Could you check a few things on this model? Use its own coordinates, in mm. Give positions to 0.01 mm unless a question says otherwise; leave off trailing zeros. Write each question's results on one line, items separated by ' | '. Start each with the question number.
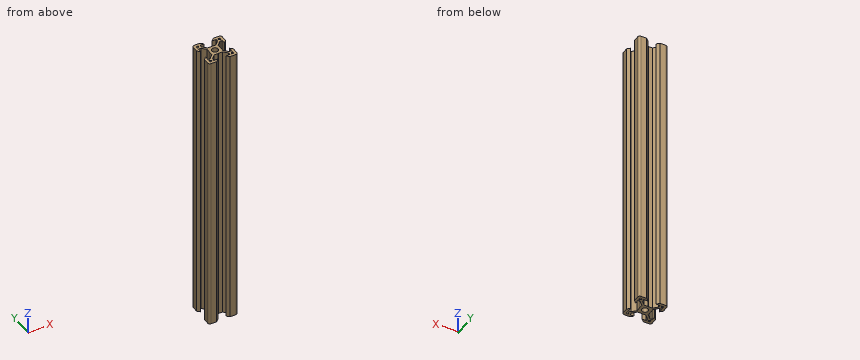
from build123d import *

# Parameters (mm, degrees)
F1_DEPTH = 200


with BuildPart() as f1:
    # F0 (on Top) → F1 (new body)
    with BuildSketch(Plane.XY):
        with BuildLine():
            Line((0, -3.729949), (0, -2.1))
            ThreePointArc((0, -2.1), (-1.484924, -1.484924), (-2.1, 0))
            Line((-2.1, 0), (-3.729949, 0))
            ThreePointArc((-3.729949, 0), (-3.759239, -0.070711), (-3.829949, -0.1))
            Line((-3.829949, -0.1), (-3.829949, -2.84))
            Line((-3.829949, -2.84), (-6.56, -5.570051))
            Line((-6.56, -5.570051), (-8.2, -5.570051))
            Line((-8.2, -5.570051), (-8.2, -2.84))
            Line((-8.2, -2.84), (-10, -4.64))
            Line((-10, -4.64), (-10, -8.5))
            ThreePointArc((-10, -8.5), (-9.56066, -9.56066), (-8.5, -10))
            Line((-8.5, -10), (-4.64, -10))
            Line((-4.64, -10), (-2.84, -8.2))
            Line((-2.84, -8.2), (-5.570051, -8.2))
            Line((-5.570051, -8.2), (-5.570051, -6.56))
            Line((-5.570051, -6.56), (-2.84, -3.829949))
            Line((-2.84, -3.829949), (-0.1, -3.829949))
            ThreePointArc((-0.1, -3.829949), (-0.070711, -3.759239), (0, -3.729949))
        make_face()
        Polygon((-7.780051, -6.640051), (-6.640051, -7.780051), (-6.640051, -8.2), (-8.2, -8.2), (-8.2, -6.640051), align=None, mode=Mode.SUBTRACT)
        with BuildLine():
            ThreePointArc((-2.1, 0), (-1.484924, 1.484924), (0, 2.1))
            Line((0, 2.1), (0, 3.729949))
            ThreePointArc((0, 3.729949), (-0.070711, 3.759239), (-0.1, 3.829949))
            Line((-0.1, 3.829949), (-2.84, 3.829949))
            Line((-2.84, 3.829949), (-5.570051, 6.56))
            Line((-5.570051, 6.56), (-5.570051, 8.2))
            Line((-5.570051, 8.2), (-2.84, 8.2))
            Line((-2.84, 8.2), (-4.64, 10))
            Line((-4.64, 10), (-8.5, 10))
            ThreePointArc((-8.5, 10), (-9.56066, 9.56066), (-10, 8.5))
            Line((-10, 8.5), (-10, 4.64))
            Line((-10, 4.64), (-8.2, 2.84))
            Line((-8.2, 2.84), (-8.2, 5.570051))
            Line((-8.2, 5.570051), (-6.56, 5.570051))
            Line((-6.56, 5.570051), (-3.829949, 2.84))
            Line((-3.829949, 2.84), (-3.829949, 0.1))
            ThreePointArc((-3.829949, 0.1), (-3.759239, 0.070711), (-3.729949, 0))
            Line((-3.729949, 0), (-2.1, 0))
        make_face()
        Polygon((-6.640051, 7.780051), (-7.780051, 6.640051), (-8.2, 6.640051), (-8.2, 8.2), (-6.640051, 8.2), align=None, mode=Mode.SUBTRACT)
        with BuildLine():
            Line((3.729949, 0), (2.1, 0))
            ThreePointArc((2.1, 0), (1.484924, -1.484924), (0, -2.1))
            Line((0, -2.1), (0, -3.729949))
            ThreePointArc((0, -3.729949), (0.070711, -3.759239), (0.1, -3.829949))
            Line((0.1, -3.829949), (2.84, -3.829949))
            Line((2.84, -3.829949), (5.570051, -6.56))
            Line((5.570051, -6.56), (5.570051, -8.2))
            Line((5.570051, -8.2), (2.84, -8.2))
            Line((2.84, -8.2), (4.64, -10))
            Line((4.64, -10), (8.5, -10))
            ThreePointArc((8.5, -10), (9.56066, -9.56066), (10, -8.5))
            Line((10, -8.5), (10, -4.64))
            Line((10, -4.64), (8.2, -2.84))
            Line((8.2, -2.84), (8.2, -5.570051))
            Line((8.2, -5.570051), (6.56, -5.570051))
            Line((6.56, -5.570051), (3.829949, -2.84))
            Line((3.829949, -2.84), (3.829949, -0.1))
            ThreePointArc((3.829949, -0.1), (3.759239, -0.070711), (3.729949, 0))
        make_face()
        Polygon((6.640051, -7.780051), (7.780051, -6.640051), (8.2, -6.640051), (8.2, -8.2), (6.640051, -8.2), align=None, mode=Mode.SUBTRACT)
        with BuildLine():
            ThreePointArc((0, 2.1), (1.484924, 1.484924), (2.1, 0))
            Line((2.1, 0), (3.729949, 0))
            ThreePointArc((3.729949, 0), (3.759239, 0.070711), (3.829949, 0.1))
            Line((3.829949, 0.1), (3.829949, 2.84))
            Line((3.829949, 2.84), (6.56, 5.570051))
            Line((6.56, 5.570051), (8.2, 5.570051))
            Line((8.2, 5.570051), (8.2, 2.84))
            Line((8.2, 2.84), (10, 4.64))
            Line((10, 4.64), (10, 8.5))
            ThreePointArc((10, 8.5), (9.56066, 9.56066), (8.5, 10))
            Line((8.5, 10), (4.64, 10))
            Line((4.64, 10), (2.84, 8.2))
            Line((2.84, 8.2), (5.570051, 8.2))
            Line((5.570051, 8.2), (5.570051, 6.56))
            Line((5.570051, 6.56), (2.84, 3.829949))
            Line((2.84, 3.829949), (0.1, 3.829949))
            ThreePointArc((0.1, 3.829949), (0.070711, 3.759239), (0, 3.729949))
            Line((0, 3.729949), (0, 2.1))
        make_face()
        Polygon((6.640051, 8.2), (8.2, 8.2), (8.2, 6.640051), (7.780051, 6.640051), (6.640051, 7.780051), align=None, mode=Mode.SUBTRACT)
    extrude(amount=F1_DEPTH)


solid = f1.part
Q1. Please list where these lines run through material, in increasing order: line 1 (Y direction, x = 8, z = 17); line 2 (Y direction, x = -0.25, z = 166); line 3 (X direction, y = -7.25, z = 166). Write a range as [from, to].
Q2. If we section it at A-A (z = 134): Count the separate pieces of the cut face and the enclosed holes in it, plus the area to 3 significant figures.
Q3. I'm going to push flat-ended pins straight in: P1, Ø3, axis at x = -5, y = -0.5, coming from the -Z side; P2, Ø0.8, axis at y = 2, z = 78.5, coming from the -X side; P3, Ø5, axis at y = -2, z = 114, coming from the -X side; P4, Ø2, axis at x = 1, z = 66.5, coming from the +Y side. Where does each tip first touch, or does it pass through?
Determined:
1) line 1: y = [-10, -8.2], [-6.64, -5.57], [5.57, 6.64], [8.2, 10] | line 2: y = [-3.83, -2.09], [2.09, 3.83] | line 3: x = [-10, -8.2], [-7.17, -5.57], [5.57, 7.17], [8.2, 10]
2) separate pieces: 1 | enclosed holes: 5 | area: 158 mm²
3) P1: stops at z = 0 | P2: stops at x = -3.83 | P3: stops at x = -9.86 | P4: stops at y = 3.83
